The model under review builds one solid part; all positions refer to its coordinate system, in mm. Coordinates: 2 decimals unless noted, no trailing zeros. Write each loop counter-clockwise with the first axis right and the second up, starting at its lowest first coordinate (ties: lowest second). Pieces come first, ordered by that corner, then holes.
1) For line 1 (Z direction, x = 0, y = -14); line 2 (Y direction, x = 19, z = 1.5); line 3 (X direction, y = 12, z = 1), list the stretches that pass through material, from the lowest coordinate up.
2) Add section B-B, the plane y = -1.5. State the section outline as (x, z) points.
3) For P1, Ø4, axis at x = 9.5, z = 7, coming from the -Y side; P2, Ø2, axis at x = -20.5, z = -2.5, coming from the +Y side; P3, Ø10, axis at x = 9, y = 121, coming from the +Z side, all flat-tipped, find the tip position at first contact; note any pin that passes through.
4) Add section A-A, the plane y = 73. State the section outline as (x, z) points.
from build123d import *

# Parameters (mm, degrees)
SKETCH1_R                 = 5
CENTERSCREW_DEPTH         = 140
SKETCH2_R                 = 3.5
TEETHWHEELCONNECTOR_DEPTH = 17
INNERHOLE_D               = 4
INNERHOLE_DEPTH           = 10
INNERHOLE_TIP             = 1.201721238
SKETCH5_R                 = 27.5
BOSS_EXTRUDE3_DEPTH       = 5
CUT_EXTRUDE5_DEPTH        = 5
CIRPATTERN1_COUNT         = 24
BOSS_EXTRUDE4_START       = 10
SKETCH10_R                = 3.5
BOSS_EXTRUDE4_DEPTH       = 10


with BuildPart() as part:
    # Sketch1 → centerScrew (new body)
    with BuildSketch(Plane(origin=(0, 0, 0), x_dir=(1, 0, 0), z_dir=(0, 1, 0))):
        with Locations(Location((0, 0, 0), (0, 0, 270))):
            Circle(SKETCH1_R)
    extrude(amount=CENTERSCREW_DEPTH)

    # Sketch2 → teethWheelConnector (add)
    with BuildSketch(Plane.XZ):
        with Locations(Location((0, 0, 0), (0, 0, 270))):
            Circle(SKETCH2_R)
    extrude(amount=TEETHWHEELCONNECTOR_DEPTH)

    # innerHole
    with Locations(Plane(origin=(0, -17, 0), x_dir=(-1, 0, 0), z_dir=(0, -1, 0))):
        with Locations((0, 0)):
            Hole(INNERHOLE_D / 2, depth=INNERHOLE_DEPTH)
            with Locations((0, 0, -(INNERHOLE_DEPTH + INNERHOLE_TIP / 2))):  # 118° drill point
                Cone(0, INNERHOLE_D / 2, INNERHOLE_TIP, mode=Mode.SUBTRACT)

    # Sketch5 → Boss-Extrude3 (add, symmetric)
    with BuildSketch(Plane(origin=(0, -8, 0), x_dir=(-1, 0, 0), z_dir=(0, -1, 0))):
        with Locations(Location((0, 0, 0), (0, 0, 90))):
            Circle(SKETCH5_R)
    extrude(amount=BOSS_EXTRUDE3_DEPTH, both=True)

    # Sketch9 → Cut-Extrude5 (cut, symmetric)
    with BuildSketch(Plane(origin=(0, -8, 0), x_dir=(-1, 0, 0), z_dir=(0, -1, 0))):
        with BuildLine():
            Line((4.013866942, 30.488346334), (0.652630961, 19.957224307))
            ThreePointArc((0.652630961, 19.957224307), (0, 20), (-0.652630961, 19.957224307))
            Line((-0.652630961, 19.957224307), (-4.013866942, 30.488346334))
            ThreePointArc((-4.013866942, 30.488346334), (0, 31), (4.013866942, 30.488346334))
        make_face()
    cut_extrude5 = extrude(amount=CUT_EXTRUDE5_DEPTH, both=True, mode=Mode.SUBTRACT)

    # CirPattern1: Cut-Extrude5 ×24 about axis
    cirpattern1_axis = Axis((0, 0, 0), (0, 1, 0))
    for i in range(1, CIRPATTERN1_COUNT):
        add(cut_extrude5.rotate(cirpattern1_axis, i * 360 / CIRPATTERN1_COUNT), mode=Mode.SUBTRACT)

    # Sketch10 → Boss-Extrude4 (add)
    with BuildSketch(Plane(origin=(0, 140, 0), x_dir=(1, 0, 0), z_dir=(0, 1, 0)).offset(BOSS_EXTRUDE4_START)):
        with Locations(Location((0, 0, 0), (0, 0, 90))):
            Circle(SKETCH10_R)
    extrude(amount=-BOSS_EXTRUDE4_DEPTH)


solid = part.part
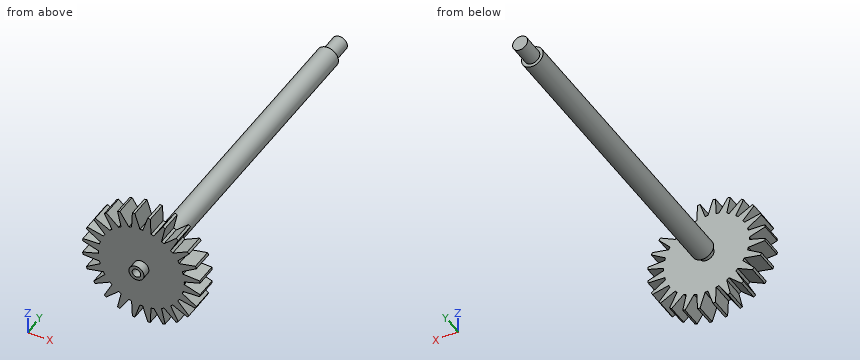
Geometry results:
1. line 1: z = -3.5 to -2, 2 to 3.5
1. line 2: y = -13 to -3
1. line 3: x = -4.9 to 4.9
2. outline: circle Ø7 at (0, 0)
3. P1: stops at y = -13
3. P2: stops at y = -3
3. P3: stops at z = 3
4. outline: circle Ø10 at (0, 0)
